```python
from build123d import *

# Parameters (mm, degrees)
SKETCH_1_W          = 96
SKETCH_1_H          = 72
EXTRUDE_1_DEPTH     = 2
SKETCH_2_W          = 24
SKETCH_2_H          = 2
CUT_EXTRUDE_1_DEPTH = 3
SKETCH_3_W          = 2
SKETCH_3_H          = 36.5
CUT_EXTRUDE_2_DEPTH = 3
SKETCH_4_W          = 2
SKETCH_4_H          = 36.5
CUT_EXTRUDE_3_DEPTH = 3


with BuildPart() as part:
    # ｽｹｯﾁ1 → ﾎﾞｽ - 押し出し1 (new body)
    with BuildSketch(Plane.XY):
        with Locations((2.027244426, 13.573770492)):
            Rectangle(SKETCH_1_W, SKETCH_1_H)
    extrude(amount=EXTRUDE_1_DEPTH)

    # ｽｹｯﾁ2 → ｶｯﾄ - 押し出し1 (cut, through all)
    with BuildSketch(Plane(origin=(0, 0, 0), x_dir=(-1, 0, 0), z_dir=(0, 0, -1))):
        with Locations((33.972755574, -21.426229508)):
            Rectangle(SKETCH_2_W, SKETCH_2_H)
        with Locations((-38.027244426, -21.426229508)):
            Rectangle(SKETCH_2_W, SKETCH_2_H)
        with Locations((33.972755574, 49.073770492)):
            Rectangle(SKETCH_2_W, SKETCH_2_H)
        with Locations((-38.027244426, 49.073770492)):
            Rectangle(SKETCH_2_W, SKETCH_2_H)
    extrude(amount=-CUT_EXTRUDE_1_DEPTH, mode=Mode.SUBTRACT)

    # ｽｹｯﾁ3 → ｶｯﾄ - 押し出し2 (cut, through all)
    with BuildSketch(Plane(origin=(0, 0, 0), x_dir=(-1, 0, 0), z_dir=(0, 0, -1))):
        with Locations((44.972755574, 13.823770492)):
            Rectangle(SKETCH_3_W, SKETCH_3_H)
    extrude(amount=-CUT_EXTRUDE_2_DEPTH, mode=Mode.SUBTRACT)

    # ｽｹｯﾁ4 → ｶｯﾄ - 押し出し3 (cut, through all)
    with BuildSketch(Plane(origin=(0, 0, 0), x_dir=(-1, 0, 0), z_dir=(0, 0, -1))):
        with Locations((-49.027244426, 13.823770492)):
            Rectangle(SKETCH_4_W, SKETCH_4_H)
    extrude(amount=-CUT_EXTRUDE_3_DEPTH, mode=Mode.SUBTRACT)


solid = part.part
```
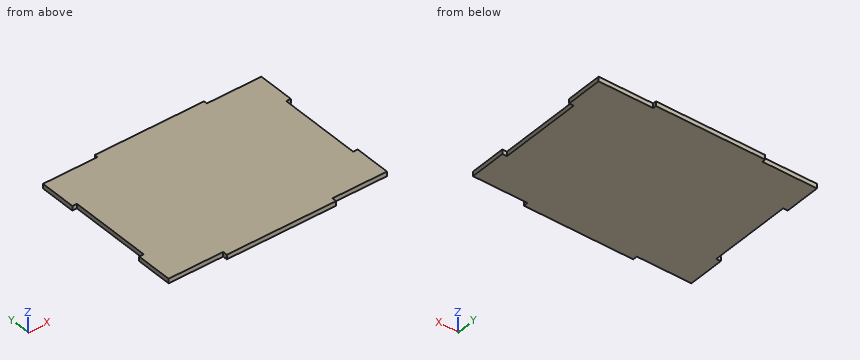
CAD build for the part. Positions are in the model's coordinates, mm. Give positions to 0.01 mm unless a question says otherwise; leave off trailing zeros. Order: outer loops, then holes, each group sorted by start corner. A loop starts at its lowest first (then second) coordinate and runs counter-clockwise, first axis right, second up.
(1) Saw through at A-A, the plane z = 0.4. Give the cut face in (x, y), then the cut area to 3 significant figures.
(2) Flat gauge pins, fed straight in: pin 1 (0.6 mm diameter, centred on x = -45, z = 0.5, fed in from -Y); pin 2 (1.2 mm diameter, centred on y = 49, z = 1, fed in from +X); pin 3 (1 mm diameter, centred on x = -34.5, z = 1.5, fed in from +Y). Where does each tip first touch, or does it go through?
(3) Drill centre lines: L1, parallel to X at y = 8, z = 0.3; L2, parallel to Y at x = -34.5, z = 1.9. Where is each one in solid material? Low to high.
(4) Saw through at C-C, the plane x = 42. Give the cut face in (y, z).
(5) Saw through at B-B, the plane y = 18.5. Give the cut face in (x, z).
Results found:
1. outline: (-45.97, -20.43) - (-21.97, -20.43) - (-21.97, -22.43) - (26.03, -22.43) - (26.03, -20.43) - (50.03, -20.43) - (50.03, -4.43) - (48.03, -4.43) - (48.03, 32.07) - (50.03, 32.07) - (50.03, 48.07) - (26.03, 48.07) - (26.03, 49.57) - (-21.97, 49.57) - (-21.97, 48.07) - (-45.97, 48.07) - (-45.97, 32.07) - (-43.97, 32.07) - (-43.97, -4.43) - (-45.97, -4.43) - close
1. area: 6,600 mm2
2. pin 1: stops at y = -20.43
2. pin 2: stops at x = 26.03
2. pin 3: stops at y = 48.07
3. L1: x = -43.97 to 48.03
3. L2: y = -20.43 to 48.07
4. outline: (-20.43, 0) - (48.07, 0) - (48.07, 2) - (-20.43, 2) - close
5. outline: (-43.97, 0) - (48.03, 0) - (48.03, 2) - (-43.97, 2) - close
